from build123d import *

# Parameters (mm, degrees)
SKETCH1_W                      = 67
SKETCH1_H                      = 40
BOSS_EXTRUDE1_DEPTH            = 32
SKETCH2_R                      = 6
CUT_EXTRUDE1_DEPTH             = 19
SKETCH4_R                      = 4
CUT_EXTRUDE2_DEPTH             = 22
LPATTERN1_COUNT                = 2
LPATTERN1_PITCH                = 45
LPATTERN1_COUNT_DIR2           = 2
LPATTERN1_PITCH_DIR2           = 14
SKETCH5_R                      = 6.5
CUT_EXTRUDE3_DEPTH             = 35
M4X0_7_TAPPED_HOLE1_D          = 3.3
CBORE_FOR_M3_SHCS1_D           = 3.4
CBORE_FOR_M3_SHCS1_CBORE_D     = 6.5
CBORE_FOR_M3_SHCS1_CBORE_DEPTH = 30
LPATTERN2_COUNT                = 2
LPATTERN2_PITCH                = 25
LPATTERN2_COUNT_DIR2           = 2
LPATTERN2_PITCH_DIR2           = 20
M3X0_5_TAPPED_HOLE1_D          = 2.5
M3X0_5_TAPPED_HOLE1_DEPTH      = 5.5
M3X0_5_TAPPED_HOLE1_TIP        = 0.751075774


with BuildPart() as part:
    # Sketch1 → Boss-Extrude1 (new body)
    with BuildSketch(Plane.XY):
        with Locations((33.5, 20)):
            Rectangle(SKETCH1_W, SKETCH1_H)
    extrude(amount=BOSS_EXTRUDE1_DEPTH)

    # Sketch2 → Cut-Extrude1 (cut)
    with BuildSketch(Plane.XZ):
        with Locations((11.5, 24.5)):
            Circle(SKETCH2_R)
    cut_extrude1 = extrude(amount=-CUT_EXTRUDE1_DEPTH, mode=Mode.SUBTRACT)

    # Sketch4 → Cut-Extrude2 (cut, through all)
    with BuildSketch(Plane.XZ.offset(-19)):
        with Locations((11.5, 24.5)):
            Circle(SKETCH4_R)
    cut_extrude2 = extrude(amount=-CUT_EXTRUDE2_DEPTH, mode=Mode.SUBTRACT)

    # LPattern1: Cut-Extrude1, Cut-Extrude2 2 × 2
    with Locations(*[(i * LPATTERN1_PITCH, 0, -j * LPATTERN1_PITCH_DIR2) for i in range(LPATTERN1_COUNT) for j in range(LPATTERN1_COUNT_DIR2) if (i, j) != (0, 0)]):
        add(cut_extrude1, mode=Mode.SUBTRACT)
        add(cut_extrude2, mode=Mode.SUBTRACT)

    # Sketch5 → Cut-Extrude3 (cut)
    with BuildSketch(Plane(origin=(0, 40, 0), x_dir=(1, 0, 0), z_dir=(0, 1, 0))):
        with Locations((33.5, -10.5)):
            Circle(SKETCH5_R)
        with Locations((33.5, -24.5)):
            Circle(SKETCH5_R)
    extrude(amount=-CUT_EXTRUDE3_DEPTH, mode=Mode.SUBTRACT)

    # M4x0.7 Tapped Hole1 (through all)
    with Locations(Plane(origin=(0, 5, 0), x_dir=(1, 0, 0), z_dir=(0, 1, 0))):
        with Locations((33.5, -24.5), (33.5, -10.5)):
            Hole(M4X0_7_TAPPED_HOLE1_D / 2)

    # CBORE for M3 SHCS1 (through all)
    with Locations(Plane.XY.offset(32)):
        with Locations((21, 30)):
            cbore_for_m3_shcs1 = CounterBoreHole(CBORE_FOR_M3_SHCS1_D / 2, CBORE_FOR_M3_SHCS1_CBORE_D / 2, CBORE_FOR_M3_SHCS1_CBORE_DEPTH)

    # LPattern2: CBORE for M3 SHCS1 2 × 2
    with Locations(*[(i * LPATTERN2_PITCH, -j * LPATTERN2_PITCH_DIR2, 0) for i in range(LPATTERN2_COUNT) for j in range(LPATTERN2_COUNT_DIR2) if (i, j) != (0, 0)]):
        add(cbore_for_m3_shcs1, mode=Mode.SUBTRACT)

    # M3x0.5 Tapped Hole1
    with Locations(Plane(origin=(0, 0, 0), x_dir=(-1, 0, 0), z_dir=(0, -1, 0))):
        with Locations((-45.5, -17.5), (-21.5, -17.5)):
            Hole(M3X0_5_TAPPED_HOLE1_D / 2, depth=M3X0_5_TAPPED_HOLE1_DEPTH)
            with Locations((0, 0, -(M3X0_5_TAPPED_HOLE1_DEPTH + M3X0_5_TAPPED_HOLE1_TIP / 2))):  # 118° drill point
                Cone(0, M3X0_5_TAPPED_HOLE1_D / 2, M3X0_5_TAPPED_HOLE1_TIP, mode=Mode.SUBTRACT)


solid = part.part
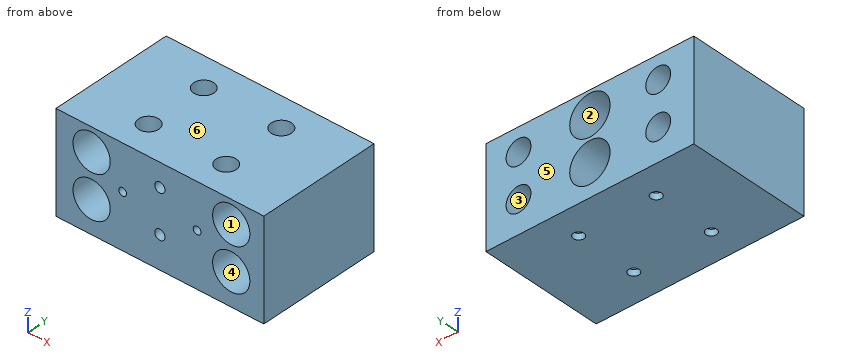
For this review, take the finished solid that the model builds, in its own axes (mm). Face numbers are marked on the shaded views. A direction names the side the tool comes from. Round coordinates to 2 decimals unless told otherwise and drop trailing zeros. Loops run counter-clockwise (first coordinate to the right, second up) from the corner with the lowest first, then second, coordinate; pieces in that order, holes last. Notation, with made-up numbers: (-28.75, -4) - (11.25, -4) arc R26 ccw to (11.25, 16) - close; hole circle Ø2 at (-8.75, 29). An arc over 180 degrees is marked (long way). Answer as CSV lines item,"result".
(1) Wall thickness on line 1 (Y direction, x = 21, z = 2.5); line 2 (Z direction, x = 33.5, y = 2.7); line 3 (X direction, y = 2.2, z = 17.5): over which ranges is each line inside the solid? List them lowest first.
Checked values:
line 1,"y = 0 to 6.75, 13.25 to 26.75, 33.25 to 40"
line 2,"z = 0 to 8.85, 12.15 to 22.85, 26.15 to 32"
line 3,"x = 0 to 20.25, 22.75 to 44.25, 46.75 to 67"
(2) Consider section A-A on z = 24.5. Give the number of separate pieces and of enclosed holes in the cut face, then the cut area to 3 significant figures.
Checked values:
separate pieces,"4"
enclosed holes,"4"
area,"1,280 mm2"
(3) Tool access review of the marked faces 1, 2 and 3: name each direction out of +Z, -Z, +X, -X, +Y, -Y from which nothing blocks a thin tool from reaching the whole face with its end or side.
Checked values:
face 1,"-Y"
face 2,"+Y"
face 3,"+Y, -Y"
(4) Insertion check: P1, Ø1, axis at x = 11, z = 13, coming from the +Y side; P2, Ø2, axis at x = 19.5, y = 9.5, coming from the +Z side; P3, Ø6, axis at x = 57, z = 12, coming from the -Y side. Each pin has a flat end and moves straight along its axis. Give the tip position at first contact, or say it passes through.
Checked values:
P1,"passes through"
P2,"stops at z = 2"
P3,"stops at y = 19"
(5) Consider section C-C on x = 56.5. Give the boundary of the cut face in (y, z).
Checked values:
outline,"(0, 0) - (40, 0) - (40, 6.5) - (19, 6.5) - (19, 4.5) - (0, 4.5) - close; (0, 16.5) - (19, 16.5) - (19, 14.5) - (40, 14.5) - (40, 20.5) - (19, 20.5) - (19, 18.5) - (0, 18.5) - close; (0, 30.5) - (19, 30.5) - (19, 28.5) - (40, 28.5) - (40, 32) - (0, 32) - close"
(6) Consider section D-D on z = 8. Give the boundary of the cut face in (x, y).
Checked values:
outline,"(0, 0) - (6.05, 0) - (6.05, 19) - (8.38, 19) - (8.38, 40) - (0, 40) - close; (14.62, 19) - (16.95, 19) - (16.95, 0) - (51.05, 0) - (51.05, 19) - (53.38, 19) - (53.38, 40) - (39.5, 40) - (39.5, 5) - (27.5, 5) - (27.5, 40) - (14.62, 40) - close; (59.62, 19) - (61.95, 19) - (61.95, 0) - (67, 0) - (67, 40) - (59.62, 40) - close; hole circle Ø6.5 at (21, 10); hole circle Ø6.5 at (21, 30); hole circle Ø6.5 at (46, 10); hole circle Ø6.5 at (46, 30)"
(7) Mouldability with a two-part tool opening along Z and no side actions: class the marked faces 4, 5 and 6 as +Z half, -Z half, draft (parallel to the pull), parting line (faces both ways), or undercut.
Checked values:
face 4,"undercut"
face 5,"draft"
face 6,"+Z half"
